Input: part model. Units: mm. Frame: model coordinates. Face numbers are marked on the shaded views. Give positions to 0.01 mm unless a question says otherwise; leave off trailing zeros. Loops run counter-clockwise (first coordinate to the right, second up) from the corner with the lowest first, then second, coordinate; pieces in that order, holes last. Notation, with made-up numbers: (26.5, -20.5) -> (52.5, -20.5) arc R20 cw to (52.5, 5.5) -> close; hole circle Ø3 at (40, -35.5). An arc over 180 degrees is marked (long way). Answer in a Markdown table with one row per item. Add a question column.
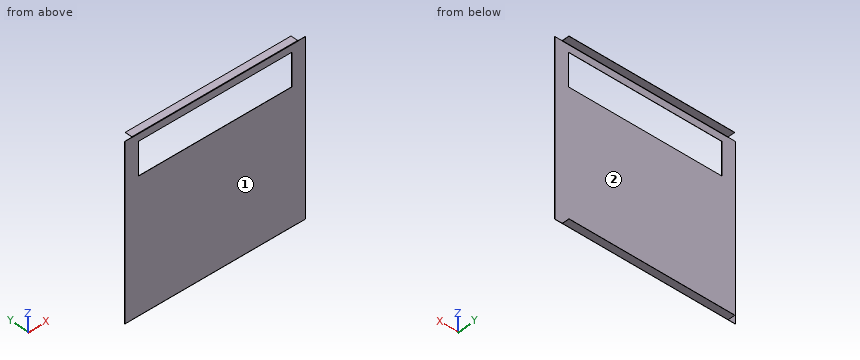
```python
from build123d import *

# Parameters (mm, degrees)
SKETCH1_W                    = 990
SKETCH1_H                    = 945
SKETCH1_W_2                  = 842
SKETCH1_H_2                  = 180
BASE_FLANGE1_DEPTH           = 1.2
EDGE_FLANGE1_STRIP_W         = 7.2
EDGE_FLANGE1_STRIP_H         = 1.2
EDGE_FLANGE1_STRIP_CUT_DEPTH = 910
EDGE_FLANGE1_DEPTH           = 910
EDGE_FLANGE2_STRIP_W         = 7.2
EDGE_FLANGE2_STRIP_H         = 1.2
EDGE_FLANGE2_STRIP_CUT_DEPTH = 910
EDGE_FLANGE2_DEPTH           = 910


# Sheet-metal steps are written as plain solids
with BuildPart() as part:
    # Sketch1 → Base-Flange1 (new body)
    with BuildSketch(Plane(origin=(0, 0, 0), x_dir=(1, 0, 0), z_dir=(0, 1, 0))):
        Rectangle(SKETCH1_W, SKETCH1_H)
        with Locations((0, -342.5)):
            Rectangle(SKETCH1_W_2, SKETCH1_H_2, mode=Mode.SUBTRACT)
    extrude(amount=-BASE_FLANGE1_DEPTH)

    # Edge-Flange1 strip (across the edge) → Edge-Flange1 strip cut (cut)
    with BuildSketch(Plane(origin=(455, 0, -472.5), x_dir=(0, 0, 1), z_dir=(-1, 0, 0))):
        with Locations((-2.4, -0.6)):
            Rectangle(EDGE_FLANGE1_STRIP_W, EDGE_FLANGE1_STRIP_H)
    extrude(amount=EDGE_FLANGE1_STRIP_CUT_DEPTH, mode=Mode.SUBTRACT)

    # Edge-Flange1 section (across the edge) → Edge-Flange1 (add)
    with BuildSketch(Plane(origin=(455, 0, -472.5), x_dir=(0, 0, 1), z_dir=(-1, 0, 0))):
        with BuildLine():
            Line((-1.2, 1.2), (-1.2, 40))
            Line((-1.2, 40), (0, 40))
            Line((0, 40), (0, 1.2))
            ThreePointArc((0, 1.2), (0.351471863, 0.351471863), (1.2, 0))
            Line((1.2, 0), (1.2, -1.2))
            ThreePointArc((1.2, -1.2), (-0.497056275, -0.497056275), (-1.2, 1.2))
        make_face()
    extrude(amount=EDGE_FLANGE1_DEPTH)

    # Edge-Flange2 strip (across the edge) → Edge-Flange2 strip cut (cut)
    with BuildSketch(Plane(origin=(-455, 0, 472.5), x_dir=(0, 0, -1), z_dir=(1, 0, 0))):
        with Locations((-2.4, -0.6)):
            Rectangle(EDGE_FLANGE2_STRIP_W, EDGE_FLANGE2_STRIP_H)
    extrude(amount=EDGE_FLANGE2_STRIP_CUT_DEPTH, mode=Mode.SUBTRACT)

    # Edge-Flange2 section (across the edge) → Edge-Flange2 (add)
    with BuildSketch(Plane(origin=(-455, 0, 472.5), x_dir=(0, 0, -1), z_dir=(1, 0, 0))):
        with BuildLine():
            Line((-1.2, 1.2), (-1.2, 40))
            Line((-1.2, 40), (0, 40))
            Line((0, 40), (0, 1.2))
            ThreePointArc((0, 1.2), (0.351471863, 0.351471863), (1.2, 0))
            Line((1.2, 0), (1.2, -1.2))
            ThreePointArc((1.2, -1.2), (-0.497056275, -0.497056275), (-1.2, 1.2))
        make_face()
    extrude(amount=EDGE_FLANGE2_DEPTH)


solid = part.part
```
1) Pull-direction query (Z, two-part tool) for the marked faces 1 and 2; classes: +Z half, -Z half, draft (parallel to the pull), parting line (faces both ways), or undercut.
2) Section A-A on x = -223.5. Output: boundary loops of the cut face in (y, z).
3) Section B-B on y = 29.5. Output: boundary loops of the cut face in (x, z), and give its area (3 significant figures).
4) Material intervals for line 1 along Z through (x, y) = (-223, 22); line 2 along Y through (x, z) = (360.5, -80), sorted ascending.
5) Section C-C on z = -20. Output: boundary loops of the cut face in (x, y), and give its area (3 significant figures).
6) Pin query (flat end, axial travel): pin 1 (1 mm diameter, centred on x = -67, y = -1, fed in from +Z); pin 2 (5 mm diameter, centred on x = -378.5, z = 82.5, fed in from +Y); pin 3 (1.9 mm diameter, centred on y = 28, z = -472.5, fed in from -X). Return the tip coordinate at first contact, or that it passes through.
Working result:
| question | item | result |
|---|---|---|
| 1 | face 1 | draft |
| 1 | face 2 | undercut |
| 2 | outline | (-1.2, -471.3) arc R2.4 ccw to (1.2, -473.7) -> (40, -473.7) -> (40, -472.5) -> (1.2, -472.5) arc R1.2 cw to (0, -471.3) -> (0, 252.5) -> (-1.2, 252.5) -> close; (-1.2, 432.5) -> (0, 432.5) -> (0, 471.3) arc R1.2 cw to (1.2, 472.5) -> (40, 472.5) -> (40, 473.7) -> (1.2, 473.7) arc R2.4 ccw to (-1.2, 471.3) -> close |
| 3 | outline | (-455, -473.7) -> (455, -473.7) -> (455, -472.5) -> (-455, -472.5) -> close; (-455, 472.5) -> (455, 472.5) -> (455, 473.7) -> (-455, 473.7) -> close |
| 3 | area | 2,180 mm2 |
| 4 | line 1 | z = -473.7 to -472.5, 472.5 to 473.7 |
| 4 | line 2 | y = -1.2 to 0 |
| 5 | outline | (-495, -1.2) -> (495, -1.2) -> (495, 0) -> (-495, 0) -> close |
| 5 | area | 1,190 mm2 |
| 6 | pin 1 | stops at z = 472.99 |
| 6 | pin 2 | stops at y = 0 |
| 6 | pin 3 | stops at x = -455 |
